Build history of the part. All positions in model axes, mm. Face numbers are marked on the shaded views. A direction names the side the tool comes from. Round coordinates to 2 decimals unless told otherwise and drop trailing zeros. Write each loop counter-clockwise with the first axis right and the second up, starting at its lowest first coordinate (ties: lowest second). Pieces come first, ordered by that corner, then holes. Notation, with made-up numbers: (-37, 1.5) - (-14, 1.5) arc R15 cw to (-14, 14.5) - close; hole circle Ø5 at (-26, -3). An arc over 180 degrees is marked (long way). Answer as a JSON object with one key per item and string values. Group by question number.
Item 1: Slice it at B-B, the plane x = 14. List the corners of the cut face in (y, z), then the cut area to 3 significant figures.
Item 2: Slice it at A-A, the plane x = 32.5. List the corners of the cut face in (y, z).
Item 3: Two-plate mould, pull along Y, no slides. Class the marked faces 1, 2, 3 and 4: +Y half, -Y half, draft (parallel to the pull), parting line (faces both ways), or undercut.
Item 4: Probe line 1 (X direction, y = -13.5, z = 8); line 2 (Y direction, x = 4.75, z = 0); line 3 (X direction, y = -16.5, z = 9). List the from-to ranges inside material, lowest first. Write a range as from..to.
Item 5: Which spindle directions (+Z, -Z, +X, -X, +Y, -Y) get a long thin tool onto all of the face, cutting with end or side? Do the marked faces 5, 6 and 7. Say none if no direction does.
Item 6: Flat gauge pins, fed straight in: pin 1 (3 mm diameter, centred on x = 67, z = 17.5, fed in from +Y); pin 2 (3 mm diameter, centred on y = 21, z = -14, fed in from +X); pin 3 (7 mm diameter, centred on y = 0, z = 0, fed in from +X); pin 4 (15 mm diameter, centred on y = -3, z = -12.5, fed in from -X). Where does each tip first touch, or does it go through?
from build123d import *


with BuildPart() as f1:
    # F0 (on Front) → F1 (revolve)
    with BuildSketch(Plane.XZ):
        with BuildLine():
            Line((0, 31), (0, 0))
            Line((0, 0), (88, 0))
            Line((88, 0), (88, 15))
            Line((88, 15), (85, 15))
            Line((85, 15), (85, 20))
            Line((85, 20), (68, 20))
            Line((68, 20), (68, 31))
            Line((68, 31), (56, 31))
            ThreePointArc((56, 31), (50, 25), (44, 31))
            Line((44, 31), (0, 31))
        make_face()
    revolve(axis=Axis((89.068668, 0, 0), (1, 0, 0)))

    # F2 (on Front) → F3 (revolve, cut)
    with BuildSketch(Plane.XZ):
        Polygon((0, 25), (0, 0), (88, 0), (88, 6), (30, 6), (30, 16), (22, 16), (22, 20.5), (15, 20.5), (15, 12.5), (12, 12.5), (12, 16), (1.5, 16), (1.5, 25), align=None)
    revolve(axis=Axis((-26.017778, 0, 0), (-1, 0, 0)), mode=Mode.SUBTRACT)


solid = f1.part
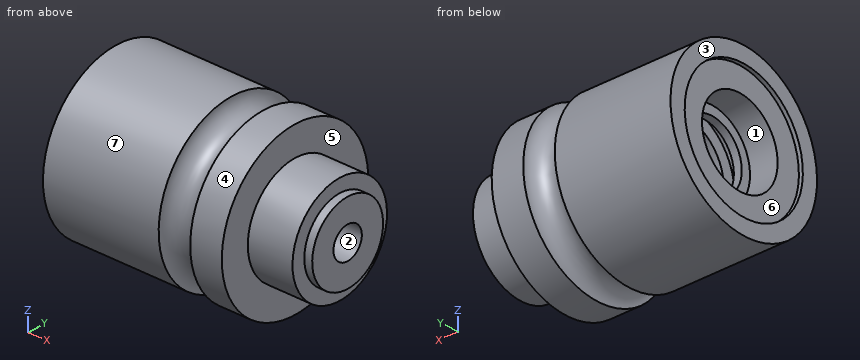
Geometry says:
{
 "1": {"outline": "circle Ø62 at (0, 0); hole circle Ø25 at (0, 0)", "area": "2,530 mm^2"},
 "2": {"outline": "circle Ø62 at (0, 0); hole circle Ø12 at (0, 0)"},
 "3": {"face 1": "undercut", "face 2": "undercut", "face 3": "draft", "face 4": "parting line"},
 "4": {"line 1": "x = 12..15, 30..85", "line 2": "y = -31..-16, 16..31", "line 3": "x = 1.5..15, 22..85"},
 "5": {"face 5": "+X", "face 6": "-X", "face 7": "+X, -X"},
 "6": {"pin 1": "stops at y = 26.55", "pin 2": "stops at x = 68", "pin 3": "passes through", "pin 4": "stops at x = 1.5"}
}
